Verification items for the finished model (mm, model axes). Face numbers are marked on the shaded views. A direction names the side the tool comes from. Give positions to 0.01 mm unless a question says otherwise; leave off trailing zeros. Write each loop counter-clockwise with the first axis right and the second up, starting at its lowest first coordinate (ties: lowest second). Pieces come first, ordered by that corner, then holes. Notation, with made-up numbers: (17, 12.25) - (36, 12.25) arc R30 cw to (36, 39.25) - close; hole circle Ø7 at (20.25, 17). An arc over 180 degrees is marked (long way). Answer as a JSON object with one key per item and string values. Group by question number.
Item 1: Sectioned sample at D-D, the plane y = 10.5. Record the boundary of the cut face in (x, z).
Item 2: Sectioned sample at C-C, the plane x = 10. Record the boundary of the cut face in (y, z).
Item 3: Go/stop test with flat-tipped pins: pin 1 (4 mm diameter, centred on y = 21, z = 24, fed in from +X); pin 2 (12 mm diameter, centred on x = 11, z = 26.5, fed in from +Y); pin 3 (2 mm diameter, centred on y = 11.5, z = 25.5, fed in from +X); pin 4 (20.5 mm diameter, centred on x = 2.41, y = 2.95, fed in from +Z). Record where each tip stops, or that it passes through.
Item 4: Scan lines: line 1 along X through (y, z) = (2.5, 25); line 2 along X through (y, z) = (-2, 13); line 3 along Y through (x, z) = (19.5, 31). Record each from-to range of solid material in increasing order. Write a range as [from, to].
Item 5: Sectioned sample at B-B, the plane y = -13. Record the boundary of the cut face in (x, z).
Item 6: Sectioned sample at A-A, the plane z = 23. Record the boundary of the cut face in (x, y), and give its area (3 significant figures).
Item 7: Draft check along X on the marked faces 3, 4, 5 and 6. Enter one of: +X half, -X half, draft (parallel to the pull), parting line (faces both ways), or undercut.
Item 8: Tool access check on the marked faces 1 and 2. Record the directions out of +Z, -Z, +X, -X, +Y, -Y that give a thin tool (end or side, any length) a straight path to the whole face; none if there is none.
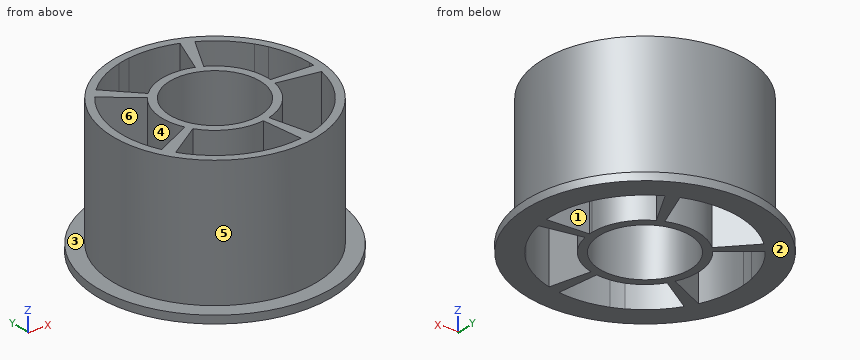
```python
from build123d import *

# Parameters (mm, degrees)
F0_R     = 26
F0_R_2   = 11.5
F1_DEPTH = 35
F0_R_3   = 30
F2_DEPTH = 2


with BuildPart() as f1:
    # F0 (on Top) → F1 (new body)
    with BuildSketch(Plane.XY):
        with Locations((2.413794294, 2.9527412442)):
            Circle(F0_R)
        with BuildLine():
            ThreePointArc((11.1447409527, 25.3082902297), (12.5504756443, 24.7069980967), (13.9150715606, 24.0174183421))
            ThreePointArc((13.9150715606, 24.0174183421), (18.7767862132, 20.5098621771), (22.6175405184, 15.9068386076))
            ThreePointArc((22.6175405184, 15.9068386076), (23.4013731254, 14.5941129329), (24.1000296021, 13.2341418376))
            ThreePointArc((24.1000296021, 13.2341418376), (25.8282091639, 8.2220083947), (26.413794294, 2.9527412442))
            ThreePointArc((26.413794294, 2.9527412442), (26.4036425051, 2.2547564238), (26.3731957266, 1.5573620862))
            ThreePointArc((26.3731957266, 1.5573620862), (26.2357288345, 0.0346194598), (26.001582844, -1.4762802416))
            ThreePointArc((26.001582844, -1.4762802416), (24.1680511465, -7.1839401061), (20.9771739376, -12.259127024))
            ThreePointArc((20.9771739376, -12.259127024), (19.9709152269, -13.410250675), (18.8934025792, -14.4949666501))
            ThreePointArc((18.8934025792, -14.4949666501), (14.0551659828, -18.0348375872), (8.4905720708, -20.2651994882))
            ThreePointArc((8.4905720708, -20.2651994882), (6.9998781675, -20.6050140543), (5.4905720708, -20.8492216688))
            ThreePointArc((5.4905720708, -20.8492216688), (-0.5043274904, -20.8691932963), (-6.3171523646, -19.4028077413))
            ThreePointArc((-6.3171523646, -19.4028077413), (-7.7228870563, -18.8015156083), (-9.0874829725, -18.1119358537))
            ThreePointArc((-9.0874829725, -18.1119358537), (-13.9491976252, -14.6043796887), (-17.7899519304, -10.0013561192))
            ThreePointArc((-17.7899519304, -10.0013561192), (-18.5758384098, -8.6849268624), (-19.2760681095, -7.3210053419))
            ThreePointArc((-19.2760681095, -7.3210053419), (-21.1447698834, -1.6291856319), (-21.5456071385, 4.3481204022))
            ThreePointArc((-21.5456071385, 4.3481204022), (-21.4081402465, 5.8708630286), (-21.173994256, 7.38176273))
            ThreePointArc((-21.173994256, 7.38176273), (-19.3404625584, 13.0894225945), (-16.1495853495, 18.1646095124))
            ThreePointArc((-16.1495853495, 18.1646095124), (-15.1433266389, 19.3157331634), (-14.0658139912, 20.4004491385))
            ThreePointArc((-14.0658139912, 20.4004491385), (-9.2275773947, 23.9403200756), (-3.6629834828, 26.1706819766))
            ThreePointArc((-3.6629834828, 26.1706819766), (-2.1722895795, 26.5104965427), (-0.6629834828, 26.7547041572))
            ThreePointArc((-0.6629834828, 26.7547041572), (5.3319160784, 26.7746757847), (11.1447409527, 25.3082902297))
        make_face(mode=Mode.SUBTRACT)
        with BuildLine():
            ThreePointArc((15.8909575998, 2.1678404678), (15.9080839128, 2.5601247827), (15.913794294, 2.9527412442))
            ThreePointArc((15.913794294, 2.9527412442), (14.0238723352, 9.8415791635), (8.8832627565, 14.8016221118))
            ThreePointArc((8.8832627565, 14.8016221118), (8.1156775536, 15.1895107237), (7.3249517895, 15.5277375486))
            ThreePointArc((7.3249517895, 15.5277375486), (-0.1658778848, 16.2039785996), (-6.8559853664, 12.7670769348))
            ThreePointArc((-6.8559853664, 12.7670769348), (-7.4620862307, 12.1569241988), (-8.0281067555, 11.5094171451))
            ThreePointArc((-8.0281067555, 11.5094171451), (-10.9856411994, 4.597468716), (-9.7875463248, -2.824566702))
            ThreePointArc((-9.7875463248, -2.824566702), (-9.3933232872, -3.5926368521), (-8.9508129572, -4.3339385227))
            ThreePointArc((-8.9508129572, -4.3339385227), (-3.2880889655, -9.2840282353), (4.1444817935, -10.4358628944))
            ThreePointArc((4.1444817935, -10.4358628944), (4.9934664729, -10.2984961112), (5.8319817935, -10.1073504178))
            ThreePointArc((5.8319817935, -10.1073504178), (12.2896748188, -6.2514417104), (15.6819253534, 0.4614166584))
            ThreePointArc((15.6819253534, 0.4614166584), (15.813632473, 1.3112977405), (15.8909575998, 2.1678404678))
        make_face()
        with Locations((2.413794294, 2.9527412442)):
            Circle(F0_R_2, mode=Mode.SUBTRACT)
        with BuildLine():
            ThreePointArc((7.3249517895, 15.5277375486), (8.1156775536, 15.1895107237), (8.8832627565, 14.8016221118))
            Line((8.8832627565, 14.8016221118), (13.9150715606, 24.0174183421))
            ThreePointArc((13.9150715606, 24.0174183421), (12.5504756443, 24.7069980967), (11.1447409527, 25.3082902297))
            Line((11.1447409527, 25.3082902297), (7.3249517895, 15.5277375486))
        make_face()
        with BuildLine():
            Line((26.3731957266, 1.5573620862), (15.8909575998, 2.1678404678))
            ThreePointArc((15.8909575998, 2.1678404678), (15.813632473, 1.3112977405), (15.6819253534, 0.4614166584))
            Line((15.6819253534, 0.4614166584), (26.001582844, -1.4762802416))
            ThreePointArc((26.001582844, -1.4762802416), (26.2357288345, 0.0346194598), (26.3731957266, 1.5573620862))
        make_face()
        with BuildLine():
            ThreePointArc((-8.0281067555, 11.5094171451), (-7.4620862307, 12.1569241988), (-6.8559853664, 12.7670769348))
            Line((-6.8559853664, 12.7670769348), (-14.0658139912, 20.4004491385))
            ThreePointArc((-14.0658139912, 20.4004491385), (-15.1433266389, 19.3157331634), (-16.1495853495, 18.1646095124))
            Line((-16.1495853495, 18.1646095124), (-8.0281067555, 11.5094171451))
        make_face()
        with BuildLine():
            Line((8.4905720708, -20.2651994882), (5.8319817935, -10.1073504178))
            ThreePointArc((5.8319817935, -10.1073504178), (4.9934664729, -10.2984961112), (4.1444817935, -10.4358628944))
            Line((4.1444817935, -10.4358628944), (5.4905720708, -20.8492216688))
            ThreePointArc((5.4905720708, -20.8492216688), (6.9998781675, -20.6050140543), (8.4905720708, -20.2651994882))
        make_face()
        with BuildLine():
            ThreePointArc((-8.9508129572, -4.3339385227), (-9.3933232872, -3.5926368521), (-9.7875463248, -2.824566702))
            Line((-9.7875463248, -2.824566702), (-19.2760681095, -7.3210053419))
            ThreePointArc((-19.2760681095, -7.3210053419), (-18.5758384098, -8.6849268624), (-17.7899519304, -10.0013561192))
            Line((-17.7899519304, -10.0013561192), (-8.9508129572, -4.3339385227))
        make_face()
    extrude(amount=F1_DEPTH)

    # F0 (on Top) → F2 (join)
    with BuildSketch(Plane.XY):
        with Locations((2.413794294, 2.9527412442)):
            Circle(F0_R_3)
        with Locations((2.413794294, 2.9527412442)):
            Circle(F0_R, mode=Mode.SUBTRACT)
    extrude(amount=F2_DEPTH)


solid = f1.part
```
Geometry check:
{
 "1": {"outline": "(-26.62, 0) - (-20.37, 0) - (-20.37, 35) - (-22.47, 35) - (-22.47, 2) - (-26.62, 2) - close; (-8.78, 0) - (-6.26, 0) - (-6.26, 35) - (-8.78, 35) - close; (11.09, 0) - (13.61, 0) - (13.61, 35) - (11.09, 35) - close; (25.2, 0) - (31.45, 0) - (31.45, 2) - (27.29, 2) - (27.29, 35) - (25.2, 35) - close"},
 "2": {"outline": "(-26.07, 0) - (-19.82, 0) - (-19.82, 35) - (-21.92, 35) - (-21.92, 2) - (-26.07, 2) - close; (-8.21, 0) - (-5.69, 0) - (-5.69, 35) - (-8.21, 35) - close; (11.6, 0) - (14.12, 0) - (14.12, 35) - (11.6, 35) - close; (16.85, 0) - (22.38, 0) - (22.38, 35) - (16.85, 35) - close; (25.72, 0) - (31.98, 0) - (31.98, 2) - (27.82, 2) - (27.82, 35) - (25.72, 35) - close"},
 "3": {"pin 1": "x = 22.87", "pin 2": "y = 28.82", "pin 3": "x = 27.29", "pin 4": "through"},
 "4": {"line 1": "[-23.58, -21.58], [-11.08, -9.08], [13.9, 15.91], [26.41, 28.41]", "line 2": "[-23.11, -21.07], [-10.14, -7.97], [12.79, 14.97], [25.9, 27.94]", "line 3": "[-16.64, -13.9], [-0.26, 1.96], [19.81, 22.55]"},
 "5": {"outline": "(-22.99, 0) - (-15.52, 0) - (-15.52, 35) - (-18.12, 35) - (-18.12, 2) - (-22.99, 2) - close; (4.48, 0) - (6.59, 0) - (6.59, 35) - (4.48, 35) - close; (20.34, 0) - (27.82, 0) - (27.82, 2) - (22.94, 2) - (22.94, 35) - (20.34, 35) - close"},
 "6": {"outline": "circle Ø52 at (2.41, 2.95); hole (-19.28, -7.32) - (-9.79, -2.82) arc R13.5 cw to (-8.03, 11.51) - (-16.15, 18.16) arc R24 ccw to start; hole (-17.79, -10) arc R24 ccw to (5.49, -20.85) - (4.14, -10.44) arc R13.5 cw to (-8.95, -4.33) - close; hole (-14.07, 20.4) - (-6.86, 12.77) arc R13.5 cw to (7.32, 15.53) - (11.14, 25.31) arc R24 ccw to start; hole circle Ø23 at (2.41, 2.95); hole (5.83, -10.11) - (8.49, -20.27) arc R24 ccw to (26, -1.48) - (15.68, 0.46) arc R13.5 cw to start; hole (8.88, 14.8) arc R13.5 cw to (15.89, 2.17) - (26.37, 1.56) arc R24 ccw to (13.92, 24.02) - close", "area": "597 mm^2"},
 "7": {"face 3": "draft", "face 4": "undercut", "face 5": "parting line", "face 6": "undercut"},
 "8": {"face 1": "+Z, -Z", "face 2": "-Z, +X, -X, +Y, -Y"}
}
